Design review of the part built by this model. Coordinates are the model's own, in mm. Face numbers are marked on the shaded views. A direction names the side the tool comes from. Give positions to 0.01 mm unless a question says otherwise; leave off trailing zeros. Order: outer loops, then holes, each group sorted by start corner. A loop starts at its lowest first (then second) coordinate and runs counter-clockwise, first axis right, second up. Notation, with made-up numbers: (24.25, 37.5) -> (74.25, 37.5) arc R6 ccw to (74.25, 48.5) -> close; hole circle Ø5 at (64, 79.25). An arc over 180 degrees is marked (long way). One line per item, written item: value.
Autodesk Inventor part; units mm, degrees
ref_plane "YZ Plane" through (0, 0, 0) normal (1, 0, 0) x (0, 1, 0)
ref_plane "XZ Plane" through (0, 0, 0) normal (0, 1, 0) x (-1, 0, 0)
ref_plane "XY Plane" through (0, 0, 0) normal (0, 0, 1) x (1, 0, 0)
sketch "Sketch1" plane through (0, 0, 0) normal (0, 1, 0) x (-1, 0, 0)
  line L0 (-10.5, 21.5) -> (-10.5, -21.5)
  line L1 (-10.5, -21.5) -> (10.5, -21.5)
  line L2 (10.5, -21.5) -> (10.5, 21.5)
  line L3 (10.5, 21.5) -> (-10.5, 21.5)
  line L4 (-10.5, 21.5) -> (10.5, -21.5) construction
  line L5 (-10.5, -21.5) -> (10.5, 21.5) construction
  point P0 (0, 0)
  dimension "d0" = 43
  dimension "d1" = 21
extrude "Extrusion1" add sketch "Sketch1" along normal blind 1.6
sketch "Sketch2" plane through (0, 1.6, 0) normal (0, 1, 0) x (1, 0, 0)
  line L0 (0, -21.5) -> (0, -17)
  line L1 (4.5, -12.5) -> (4.5, -21.5)
  line L2 (4.5, -21.5) -> (-4.5, -21.5)
  line L3 (-4.5, -21.5) -> (-4.5, -12.5)
  line L4 (-4.5, -12.5) -> (4.5, -12.5)
  line L5 (4.5, -12.5) -> (-4.5, -21.5) construction
  line L6 (4.5, -21.5) -> (-4.5, -12.5) construction
  line L7 (-2.2008, 0) -> (2.1177, 0)
  line L8 (4.5, 12.5) -> (4.5, 21.5)
  line L9 (4.5, 21.5) -> (-4.5, 21.5)
  line L10 (-4.5, 21.5) -> (-4.5, 12.5)
  line L11 (-4.5, 12.5) -> (4.5, 12.5)
  point P0 (0, 0)
  dimension "d4" = 4.5
  dimension "d5" = 9
extrude "Extrusion2" add sketch "Sketch2" along normal blind 1
sketch "Sketch3" plane through (0, 2.6, 0) normal (0, 1, 0) x (1, 0, 0)
  circle A0 centre (0, -17) radius 4
  circle A1 centre (0, 17) radius 4
  point P0 (0, 0)
  dimension "d8" = 8
  dimension "d9" = 8
extrude "Extrusion3" add sketch "Sketch3" along normal blind 10
fillet "Fillet1" radius 0.5 2 edges at (-4, 12.6, 17) (-4, 12.6, -17)
sketch "Sketch4" plane through (0, 1.6, 0) normal (0, 1, 0) x (1, 0, 0)
  line L0 (-10.5, 21.5) -> (-10.5, -21.5)
  line L1 (-10.5, -21.5) -> (-10.5, -16.5)
  line L2 (-10.5, -16.5) -> (-9.5, -16.5)
  line L3 (-9.5, -16.5) -> (-7.9, -16.5)
  line L4 (10.5, 21.5) -> (4.5, 21.5)
  line L5 (10.5, 21.5) -> (10.5, 16.5)
  line L6 (10.5, -21.5) -> (10.5, 21.5)
  line L7 (10.5, 16.5) -> (9.5, 16.5)
  line L8 (9.5, 16.5) -> (7.9, 16.5)
  point P0 (0, 0)
  dimension "d13" = 5
  dimension "d14" = 1
  dimension "d15" = 1.6
  dimension "d16" = 5
  dimension "d17" = 1
  dimension "d18" = 1.6
hole "Hole1" at (-7.9, 1.6, 16.5) at (7.9, 1.6, -16.5) direction (0, -1, 0) diameter 3.2 end through all
fillet "Fillet2" radius 1 8 edges at (4.5, 2.1, 12.5) (4.5, 2.1, -12.5) (-4.5, 2.1, -12.5) (4.5, 2.1, -21.5) (4.5, 2.1, 21.5) (-4.5, 2.1, 21.5) (-4.5, 2.1, 12.5) (-4.5, 2.1, -21.5)
properties part number "XTW-SY-8"
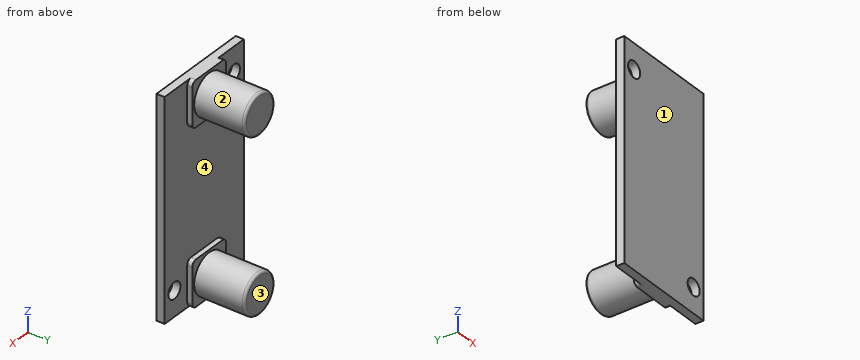
Item 1: Machinability: for the marked faces 1 and 2, which of the approach directions +Z, -Z, +X, -X, +Y, -Y give a long, thin tool a straight path to every point of the face, cutting with its end or side? Answer none if there is none.
Returned:
face 1: +Z, -Z, +X, -X, -Y
face 2: +Y
Item 2: Draft analysis for pull direction Z (two halves, no side actions). For the marked faces 3 and 4, state which applies: pulls with the +Z half, pulls with the -Z half, needs draft (parallel to the pull), parting line crosses it, or undercut.
Returned:
face 3: needs draft
face 4: undercut
Item 3: Add section C-C on y = 8.5. Give the boundary of the cut face in (x, z).
Returned:
outline: circle Ø8 at (0, -17); circle Ø8 at (0, 17)
Item 4: Add section A-A on x = -7. Give the boundary of the cut face in (y, z).
Returned:
outline: (0, -21.5) -> (1.6, -21.5) -> (1.6, 15.18) -> (0, 15.18) -> close; (0, 17.82) -> (1.6, 17.82) -> (1.6, 21.5) -> (0, 21.5) -> close
Item 5: To check wall thickness, follow line 1 along Z through (x, y) = (7.9, 1.1); line 2 along Z through (x, y) = (-7.9, 0.95); line 3 along X through (y, z) = (0.35, -16.5). State the ranges of each line that lie inside material, in increasing order. Write a range as from..to.
Returned:
line 1: -21.5..-18.1, -14.9..21.5
line 2: -21.5..14.9, 18.1..21.5
line 3: -10.5..6.3, 9.5..10.5
Item 6: Clearance check with flat-ended pins moving along their axes: P1, Ø5, axis at x = -7.9, z = 16.5, coming from the +Y side; P2, Ø2, axis at x = 0, y = 5, coming from the +Z side; P3, Ø0.5, axis at y = 2, z = 18.5, coming from the -X side. State where each tip first meets the part, or that it passes through.
Returned:
P1: y = 1.6
P2: z = 21
P3: x = -4.5
Item 7: Add section B-B on z = 17. Give the boundary of the cut face in (x, y).
Returned:
outline: (-10.5, 0) -> (-9.42, 0) -> (-9.42, 1.6) -> (-10.5, 1.6) -> close; (-6.38, 0) -> (10.5, 0) -> (10.5, 1.6) -> (4.5, 1.6) -> (4.5, 2.6) -> (4, 2.6) -> (4, 12.1) arc R0.5 ccw to (3.5, 12.6) -> (-3.5, 12.6) arc R0.5 ccw to (-4, 12.1) -> (-4, 2.6) -> (-4.5, 2.6) -> (-4.5, 1.6) -> (-6.38, 1.6) -> close
Item 8: Add section D-D on x = 0. Give the boundary of the cut face in (y, z).
Returned:
outline: (0, -21.5) -> (2.6, -21.5) -> (2.6, -21) -> (12.1, -21) arc R0.5 ccw to (12.6, -20.5) -> (12.6, -13.5) arc R0.5 ccw to (12.1, -13) -> (2.6, -13) -> (2.6, -12.5) -> (1.6, -12.5) -> (1.6, 12.5) -> (2.6, 12.5) -> (2.6, 13) -> (12.1, 13) arc R0.5 ccw to (12.6, 13.5) -> (12.6, 20.5) arc R0.5 ccw to (12.1, 21) -> (2.6, 21) -> (2.6, 21.5) -> (0, 21.5) -> close
